Input: part model. Units: mm. Frame: model coordinates. Face numbers are marked on the shaded views. A direction names the side the tool comes from. Coordinates: 2 decimals unless noted, no trailing zeros. Loops run counter-clockwise (first coordinate to the right, second up) from the corner with the lowest first, then second, coordinate; pieces in that order, holes last.
Item 1: Section A-A on z = 3. Return loops of the section in (x, y).
Item 2: Ray query, line 1 along Z through (x, y) = (2.5, 1.05); line 2 along X through (y, z) = (1.45, 2.5); line 3 along Z through (x, y) = (-1.25, 0.45). Return the intervals inside material, ascending.
Item 3: Section C-C on x = -0.25. Return loops of the section in (y, z), and give its area (3 significant figures).
Item 4: Section B-B on y = 0.75. Return loops of the section in (x, z).
Item 5: Reachability of the marked faces 1 and 2 from +Z, -Z, +X, -X, +Y, -Y: full face, straight path, thin tool, end or side. Return the list, or none.
Item 6: Pull-direction query (X, two-part tool) for the marked faces 3, 4, 5 and 6; classes: released by +X, released by -X, zero draft, split by the parting line, or undercut.
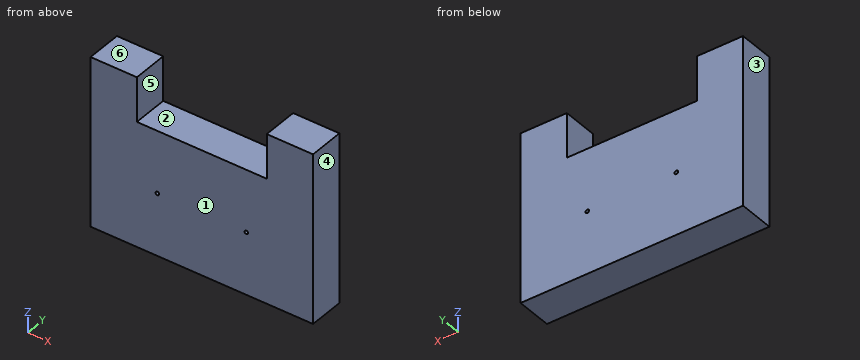
Autodesk Inventor part; units mm, degrees
ref_plane "YZ Plane" through (0, 0, 0) normal (1, 0, 0) x (0, 1, 0)
ref_plane "XZ Plane" through (0, 0, 0) normal (0, 1, 0) x (-1, 0, 0)
ref_plane "XY Plane" through (0, 0, 0) normal (0, 0, 1) x (1, 0, 0)
sketch "Sketch1" plane through (0, 0, 0) normal (0, 1, 0) x (-1, 0, 0)
  line L0 (6.25, 4.75) -> (3.65, 4.75)
  line L1 (-3.65, 4.75) -> (-6.25, 4.75)
  line L2 (6.25, 4.75) -> (6.25, -4.75)
  line L3 (6.25, -4.75) -> (-6.25, -4.75)
  line L4 (-6.25, -4.75) -> (-6.25, 4.75)
  circle A0 centre (2.5, -1.25) radius 0.1
  circle A1 centre (-2.5, -1.25) radius 0.1
  line L5 (3.65, 4.75) -> (3.65, 2.25)
  line L6 (3.65, 2.25) -> (-3.65, 2.25)
  line L7 (-3.65, 2.25) -> (-3.65, 4.75)
  dimension "d0" = 12.5
  dimension "d1" = 9.5
  dimension "d2" = 2.6
  dimension "d7" = 0.2
  dimension "d9" = 0.2
  dimension "d17" = 2.6
  dimension "d18" = 2.5
  dimension "d19" = 7.3
extrude "Extrusion1" add sketch "Sketch1" along normal blind 2
properties part number "PCB_kon_drzak"
Results found:
1. outline: (-6.25, 0) - (-3.65, 0) - (-3.65, 2) - (-6.25, 2) - close; (3.65, 0) - (6.25, 0) - (6.25, 2) - (3.65, 2) - close
2. line 1: z = -4.75 to -1.35, -1.15 to 2.25
2. line 2: x = -6.25 to -3.65, 3.65 to 6.25
2. line 3: z = -4.75 to 2.25
3. outline: (0, -4.75) - (2, -4.75) - (2, 2.25) - (0, 2.25) - close
3. area: 14.0 mm2
4. outline: (-6.25, -4.75) - (6.25, -4.75) - (6.25, 4.75) - (3.65, 4.75) - (3.65, 2.25) - (-3.65, 2.25) - (-3.65, 4.75) - (-6.25, 4.75) - close; hole circle Ø0.2 at (-2.5, -1.25); hole circle Ø0.2 at (2.5, -1.25)
5. face 1: +Z, -Z, +X, -X, -Y
5. face 2: +Z, +Y, -Y
6. face 3: released by -X
6. face 4: released by +X
6. face 5: undercut
6. face 6: zero draft
